The listing builds one solid part. Answer for the finished solid, in the listing's coordinates (mm). Face numbers are marked on the shaded views. A direction names the side the tool comes from. Coordinates: 2 decimals unless noted, no trailing zeros. Order: outer loops, then holes, each group sorted by start corner. A loop starts at its lowest first (then second) coordinate and runs counter-clockwise, first axis right, second up. Notation, with made-up numbers: (40.5, 73) - (67.5, 73) arc R27 ccw to (67.5, 103) - close; hole circle Ø3 at (53.25, 53). An arc over 180 degrees is marked (long way). One line per item, written item: value. Start each with the question number.
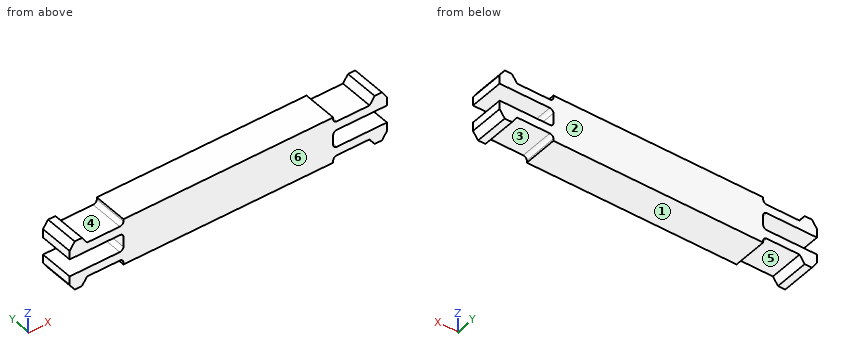
```python
from build123d import *

# Parameters (mm, degrees)
SKETCH1_W            = 57.6
SKETCH1_H            = 12.7
BOSS_EXTRUDE1_DEPTH  = 9.525
BOSS_EXTRUDE2_DEPTH  = 9.525
MIRROR2_COPY_1_DEPTH = 9.525
FILLET1_R            = 1


with BuildPart() as part:
    # Sketch1 → Boss-Extrude1 (new body)
    with BuildSketch(Plane(origin=(0, 0, 0), x_dir=(1, 0, 0), z_dir=(0, 1, 0))):
        Rectangle(SKETCH1_W, SKETCH1_H)
    extrude(amount=BOSS_EXTRUDE1_DEPTH)

    # Sketch2 → Boss-Extrude2 (add)
    with BuildSketch(Plane(origin=(0, 9.525, 0), x_dir=(1, 0, 0), z_dir=(0, 1, 0))):
        Polygon((-28.8, 4.7625), (-38.8, 4.7625), (-40.189474334, 6.746875), (-42.189474334, 6.746875), (-43.578948667, 4.7625), (-43.578948667, 2.38125), (-28.8, 2.38125), align=None)
    boss_extrude2 = extrude(amount=-BOSS_EXTRUDE2_DEPTH)

    # Mirror1: Boss-Extrude2 across plane
    add(boss_extrude2.mirror(Plane(origin=(0, 0, 0), x_dir=(0, 0, 1), z_dir=(1, 0, 0))))

    # Mirror2: Boss-Extrude2 across plane
    add(boss_extrude2.mirror(Plane.XY))

    # Mirror2 copy 1 sketch → Mirror2 copy 1 (add)
    with BuildSketch(Plane(origin=(0, 9.525, 0), x_dir=(-1, 0, 0), z_dir=(0, 1, 0))):
        Polygon((-28.8, 4.7625), (-38.8, 4.7625), (-40.189474334, 6.746875), (-42.189474334, 6.746875), (-43.578948667, 4.7625), (-43.578948667, 2.38125), (-28.8, 2.38125), align=None)
    extrude(amount=-MIRROR2_COPY_1_DEPTH)

    # Fillet1
    fillet1_edges = [part.edges().sort_by_distance(p)[0] for p in [
        (-28.8, 4.7625, -4.7625),
        (-28.8, 4.7625, -2.38125),
        (28.8, 4.7625, -4.7625),
        (28.8, 4.7625, -2.38125),
        (-28.8, 4.7625, 4.7625),
        (-28.8, 4.7625, 2.38125),
        (28.8, 4.7625, 4.7625),
        (28.8, 4.7625, 2.38125),
    ]]
    fillet(fillet1_edges, radius=FILLET1_R)


solid = part.part
```
(1) Flat-ended cylindrical pins translate along their axes: pin 1 Ø5 at (x, y) = (3, 4.5) entering from -Z; pin 2 Ø5 at (x, y) = (7, 2.5) entering from +Z; pin 3 Ø3 at (x, y) = (34, 4) entering from +Z. Find the tip coordinate at first contact, or state that the pin passes through.
(2) For a pull along X with two mould halves and no side action, classify the marked faces 1, 2 and 3 as pulls with the +X half, pulls with the -X half, needs draft (parallel to the pull), parting line crosses it, or undercut.
(3) The part is cut by section A-A on x = -33. Determine the outline of the cut face in (y, z) (1 decimal), plus the area to 3 significant figures.
(4) For the marked faces 4, 5 and 6, determine the directions among +Z, -Z, +X, -X, +Y, -Y from which every point of the face is accessible in a straight line to the end or side of a thin tool.
(5) Consider probe 1 along Z at (x, y) = (-31.5, 6.75); probe 2 along Z at (x, y) = (40.5, 7.75); probe 3 along X at (y, z) = (2, -1.5). Determine where each line is inside the solid, lowest interval first.
(6) The part is cut by section B-B on x = 15.5. Determine the outline of the cut face in (y, z) (3 decimals).
Completed:
1. pin 1: stops at z = -6.35
1. pin 2: stops at z = 6.35
1. pin 3: stops at z = 4.76
2. face 1: undercut
2. face 2: needs draft
2. face 3: undercut
3. outline: (0, -4.8) - (9.5, -4.8) - (9.5, -2.4) - (0, -2.4) - close; (0, 2.4) - (9.5, 2.4) - (9.5, 4.8) - (0, 4.8) - close
3. area: 45.4 mm2
4. face 4: +Z, +Y, -Y
4. face 5: -Z, +Y, -Y
4. face 6: +Z, -Z, +X, -X, -Y
5. probe 1: z = -4.76 to -2.38, 2.38 to 4.76
5. probe 2: z = -6.75 to -2.38, 2.38 to 6.75
5. probe 3: x = -28.81 to 28.81
6. outline: (0, -6.35) - (9.525, -6.35) - (9.525, 6.35) - (0, 6.35) - close
